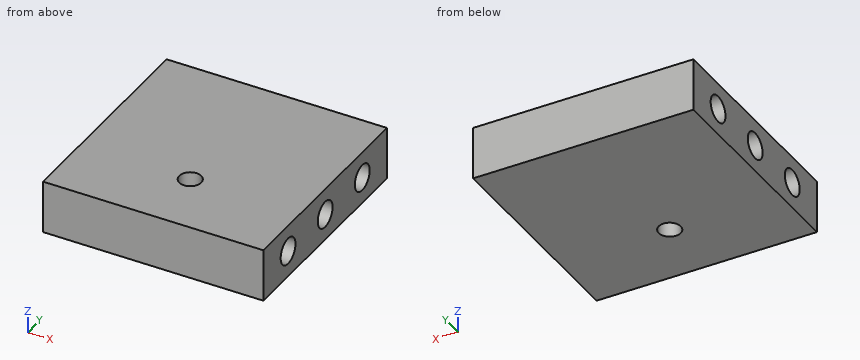
```python
from build123d import *

# Parameters (mm, degrees)
F0_W     = 50
F0_H     = 50
F1_DEPTH = 12
F2_R     = 3
F3_DEPTH = 15
F4_R     = 3
F5_DEPTH = 15
F6_R     = 3
F7_DEPTH = 50.001
F8_R     = 2.5
F9_DEPTH = 12.001


with BuildPart() as f1:
    # F0 (on Top) → F1 (new body)
    with BuildSketch(Plane.XY):
        with Locations((-5.501713, -4.568746)):
            Rectangle(F0_W, F0_H)
    extrude(amount=F1_DEPTH)

    # F2 (on face) → F3 (cut)
    with BuildSketch(Plane(origin=(-30.501713, 0, 0), x_dir=(0, -1, 0), z_dir=(-1, 0, 0))):
        with Locations((-10.431254, 6)):
            Circle(F2_R)
        with Locations((19.568746, 6)):
            Circle(F2_R)
    extrude(amount=-F3_DEPTH, mode=Mode.SUBTRACT)

    # F4 (on face) → F5 (cut)
    with BuildSketch(Plane.YZ.offset(19.498287)):
        with Locations((10.431254, 6)):
            Circle(F4_R)
        with Locations((-19.568746, 6)):
            Circle(F4_R)
    extrude(amount=-F5_DEPTH, mode=Mode.SUBTRACT)

    # F6 (on face) → F7 (cut, through all)
    with BuildSketch(Plane.YZ.offset(19.498287)):
        with Locations((-4.568746, 6)):
            Circle(F6_R)
    extrude(amount=-F7_DEPTH, mode=Mode.SUBTRACT)

    # F8 (on face) → F9 (cut, through all)
    with BuildSketch(Plane(origin=(0, 0, 0), x_dir=(1, 0, 0), z_dir=(0, 0, -1))):
        with Locations((-5.501713, 14.568746)):
            Circle(F8_R)
    extrude(amount=-F9_DEPTH, mode=Mode.SUBTRACT)


solid = f1.part
```
Here's how the part is built. I have some questions about the finished solid (model axes, mm). Round coordinates to 2 decimals unless told otherwise and drop trailing zeros. Loops run counter-clockwise (first coordinate to the right, second up) from the corner with the lowest first, then second, coordinate; pieces in that order, holes last. Notation, with made-up numbers: (40, -28) -> (51, -28) arc R15 ccw to (51, -8) -> close; hole circle Ø6 at (5, 2). An arc over 180 degrees is marked (long way). Answer as CSV lines item,"result". Start each with the question number.
1. Imagine slicing it at B-B on x = -2. Write out the boundary of the cut face in (y, z), plus the area to 3 significant figures.
2. I'm going to push flat-ended pins straight in: P1, Ø3, axis at y = 9, z = 6, coming from the +X side; P2, Ø5.5, axis at y = 10.43, z = 6, coming from the -X side. Where does each tip first touch, or does it pass through?
3. I need wall thicknesses on probe 1 along Y at (x, z) = (13, 7); probe 2 along X at (y, z) = (-20.5, 7.75); probe 3 along Y at (x, z) = (-7.5, 8). Which ranges of each line are inside material? Lowest first, please. Write a range as from..to.
4. Imagine slicing it at A-A on z = 5.25. Write out the boundary of the cut face in (x, y), plus the area to 3 significant figures.
Solution:
1,outline,"(-29.57, 0) -> (20.43, 0) -> (20.43, 12) -> (-29.57, 12) -> close; hole circle Ø6 at (-4.57, 6)"
1,area,"572 mm²"
2,P1,"x = 4.5"
2,P2,"x = -15.5"
3,probe 1,"-29.57..-22.4, -16.74..-7.4, -1.74..7.6, 13.26..20.43"
3,probe 2,"-15.5..4.5"
3,probe 3,"-29.57..-16.07, -13.07..-6.8, -2.33..20.43"
4,outline,"(-30.5, -29.57) -> (19.5, -29.57) -> (19.5, -22.47) -> (4.5, -22.47) -> (4.5, -16.66) -> (19.5, -16.66) -> (19.5, -7.47) -> (-30.5, -7.47) -> (-30.5, -16.66) -> (-15.5, -16.66) -> (-15.5, -22.47) -> (-30.5, -22.47) -> close; (-30.5, -1.66) -> (19.5, -1.66) -> (19.5, 7.53) -> (4.5, 7.53) -> (4.5, 13.34) -> (19.5, 13.34) -> (19.5, 20.43) -> (-30.5, 20.43) -> (-30.5, 13.34) -> (-15.5, 13.34) -> (-15.5, 7.53) -> (-30.5, 7.53) -> close; hole circle Ø5 at (-5.5, -14.57)"
4,area,"1,840 mm²"
